Model file for the job. Use its own axes, mm. Round coordinates to 2 decimals unless told otherwise and drop trailing zeros. Loops run counter-clockwise (first coordinate to the right, second up) from the corner with the lowest first, then second, coordinate; pieces in that order, holes last. Notation, with made-up numbers: (65, 86) - (91, 86) arc R31 cw to (91, 122) - close; hole circle Ø6 at (20.25, 60). An arc over 180 degrees is marked (long way). Use one line per item in the form item = value.
from build123d import *

# Parameters (mm, degrees)
F0_W     = 152.4
F0_H     = 127
F0_R     = 0.79375
F1_DEPTH = 6.35
F3_D     = 3.7973
F5_D     = 3.7973
F8_D     = 4.4958


with BuildPart() as f1:
    # F0 (on Front) → F1 (new body)
    with BuildSketch(Plane.XZ):
        Rectangle(F0_W, F0_H)
        Circle(F0_R, mode=Mode.SUBTRACT)
    extrude(amount=F1_DEPTH)

    # F3 (through all)
    with Locations(Plane(origin=(0, 0, 0), x_dir=(-1, 0, 0), z_dir=(0, 1, 0))):
        with Locations((0, 33.7693), (33.7693, 0), (-33.7693, 0), (0, -33.7693)):
            Hole(F3_D / 2)

    # F5 (through all)
    with Locations(Plane(origin=(0, 0, 0), x_dir=(-1, 0, 0), z_dir=(0, 1, 0))):
        with Locations((0, 53.975), (60.325, 0), (0, -53.975), (-60.325, 0)):
            Hole(F5_D / 2)

    # F8 (through all)
    with Locations(Plane.XZ.offset(6.35)):
        with Locations((-60.96, -44.45), (60.96, -44.45)):
            Hole(F8_D / 2)


solid = f1.part
1. Pull direction Z, two halves, no side cores. Call faces 1 (the cylindrical face through (-0.41, -3.22, -55.83)), 2 (the flat face through (-1, -3, 63.5)), 3 (the cylindrical face through (-58.514, -3.219, 0.57)), 4 (the flat face through (-1, -3, -63.5)): +Z half, -Z half, draft (parallel to the pull), parting line (faces both ways), or undercut.
Geometry check:
face_1 = undercut
face_2 = +Z half
face_3 = undercut
face_4 = -Z half
2. Wall check: probe 1 along Z at (x, y) = (61.5, -2.25); probe 2 along Z at (x, y) = (-60.96, -4.25); probe 3 along Z at (x, y) = (-1.5, -2). Give the ranges that are in metal, low to high.
Geometry check:
probe_1 = -63.5 to -46.63, -42.27 to -1.49, 1.49 to 63.5
probe_2 = -63.5 to -46.7, -42.2 to -1.79, 1.79 to 63.5
probe_3 = -63.5 to -55.14, -52.81 to -34.93, -32.61 to 32.61, 34.93 to 52.81, 55.14 to 63.5
3. Cut at A-A, the plane z = -44.45. Give the cut face in (x, y), plus the area to 3 significant figures.
Geometry check:
outline = (-76.2, -6.35) - (-63.21, -6.35) - (-63.21, 0) - (-76.2, 0) - close; (-58.71, -6.35) - (58.71, -6.35) - (58.71, 0) - (-58.71, 0) - close; (63.21, -6.35) - (76.2, -6.35) - (76.2, 0) - (63.21, 0) - close
area = 911 mm^2
